CAD build for the part. Positions are in the model's coordinates, mm. A direction names the side the tool comes from. Round coordinates to 2 decimals unless told otherwise and drop trailing zeros. Order: outer loops, then holes, each group sorted by start corner. A loop starts at its lowest first (then second) coordinate and runs counter-clockwise, first axis right, second up. Notation, with made-up numbers: (31.5, 69.5) -> (85.5, 69.5) arc R22 cw to (85.5, 99.5) -> close; hole circle Ø3 at (76, -18.5). An arc over 180 degrees is marked (long way). Return JSON: item names as keys, results as strings. Group by question number.
Q1. Flat gauge pins, fed straight in: pin 1 (1.8 mm diameter, centred on x = 3.5, z = 2, fed in from +Y); pin 2 (1.8 mm diameter, centred on y = -45.5, z = 3, fed in from +X); pin 3 (1.8 mm diameter, centred on y = -25.5, z = 3.5, fed in from -X). Where does each tip first touch, or does it go through?
Q2. Mould opens along Y. For faces 4 (the flat face through (189, 0, 3)), 5 (the flat face through (3, -80, 3)), 6 (the flat face through (189, -70, 3)), 7 (the flat face through (0, -55, 3)) say: +Y half, -Y half, draft (parallel to the pull), parting line (faces both ways), or undercut.
Q3. Which spindle directions (+Z, -Z, +X, -X, +Y, -Y) get a long thin tool onto all of the face, cutting with end or side? Do faces 1 (the flat face through (0, 5, 3)), 2 (the flat face through (186, -45, 3)), 3 (the flat face through (6, -65, 3)). Say none if no direction does.
Q4. Probe line 1 along X through (y, z) = (-28, 5.65). List the from-to ranges inside material, lowest first.
Q5. Cut at A-A (y = -67). Write the cut outline in (x, z), then the cut area to 3 significant figures.
Autodesk Inventor part; units mm, degrees
ref_plane "YZ Plane" through (0, 0, 0) normal (1, 0, 0) x (0, 1, 0)
ref_plane "XZ Plane" through (0, 0, 0) normal (0, 1, 0) x (-1, 0, 0)
ref_plane "XY Plane" through (0, 0, 0) normal (0, 0, 1) x (1, 0, 0)
sketch "Эскиз1" plane through (0, 0, 0) normal (0, 0, 1) x (1, 0, 0)
  line L0 (0, 0) -> (0, 10)
  line L1 (0, 0) -> (6, 0)
  line L2 (6, 10) -> (6, 0)
  line L3 (0, 10) -> (6, 10)
  line L4 (0, -20) -> (0, -10)
  line L5 (0, -20) -> (6, -20)
  line L6 (6, -10) -> (6, -20)
  line L7 (0, -10) -> (6, -10)
  line L8 (0, -40) -> (0, -30)
  line L9 (0, -40) -> (6, -40)
  line L10 (6, -30) -> (6, -40)
  line L11 (0, -30) -> (6, -30)
  line L12 (0, -60) -> (0, -50)
  line L13 (0, -60) -> (6, -60)
  line L14 (6, -50) -> (6, -60)
  line L15 (0, -50) -> (6, -50)
  line L16 (0, -80) -> (0, -70)
  line L17 (0, -80) -> (6, -80)
  line L18 (6, -70) -> (6, -80)
  line L19 (0, -70) -> (6, -70)
  line L20 (6, 22.5234) -> (6, 9.9924)
  line L21 (6, -80) -> (6, -90)
  line L22 (186, 9.9924) -> (186, 22.5234)
  line L23 (186, 0) -> (186, 10)
  line L24 (186, 0) -> (192, 0)
  line L25 (192, 10) -> (192, 0)
  line L26 (186, 10) -> (192, 10)
  line L27 (186, -20) -> (186, -10)
  line L28 (186, -20) -> (192, -20)
  line L29 (192, -10) -> (192, -20)
  line L30 (186, -10) -> (192, -10)
  line L31 (186, -40) -> (186, -30)
  line L32 (186, -40) -> (192, -40)
  line L33 (192, -30) -> (192, -40)
  line L34 (186, -30) -> (192, -30)
  line L35 (186, -60) -> (186, -50)
  line L36 (186, -60) -> (192, -60)
  line L37 (192, -50) -> (192, -60)
  line L38 (186, -50) -> (192, -50)
  line L39 (186, -80) -> (186, -70)
  line L40 (186, -80) -> (192, -80)
  line L41 (192, -70) -> (192, -80)
  line L42 (186, -70) -> (192, -70)
  line L43 (186, -90) -> (186, -80)
  line L44 (186, 22.5234) -> (6, 22.5234)
  line L45 (6, 22.5234) -> (6, -90)
  line L46 (6, -90) -> (186, -90)
  line L47 (186, -90) -> (186, 22.5234)
extrude "Выдавливание1" add sketch "Эскиз1" along normal blind 6
properties part number "полуверх"
Solution:
{
 "1": {"pin 1": "stops at y = 10", "pin 2": "stops at x = 186", "pin 3": "stops at x = 6"},
 "2": {"face 4": "undercut", "face 5": "-Y half", "face 6": "undercut", "face 7": "draft"},
 "3": {"face 1": "+Z, -Z, -X, +Y, -Y", "face 2": "+Z, -Z, +X", "face 3": "+Z, -Z, -X"},
 "4": {"line 1": "x = 6 to 186"},
 "5": {"outline": "(6, 0) -> (186, 0) -> (186, 6) -> (6, 6) -> close", "area": "1,080 mm²"}
}
